Part print with two shaded views. Sizes in mm from the minimum x, y, z corner. A direction names the side the tool comes from. Round coordinates to 2 decimals unless told otherwise and drop trailing zeros. Order: outer loops, then holes, each group sorted by start corner. A loop starts at its lowest first (then second) coordinate and runs counter-clockwise, first axis right, second up. Notation, with made-up numbers: M -40,73 L -9,73 A15 ccw -9,91 Z; hole C -2.5,2 d8. An arc over 180 degrees is marked long. Answer as a JSON object with one key per item and string values.
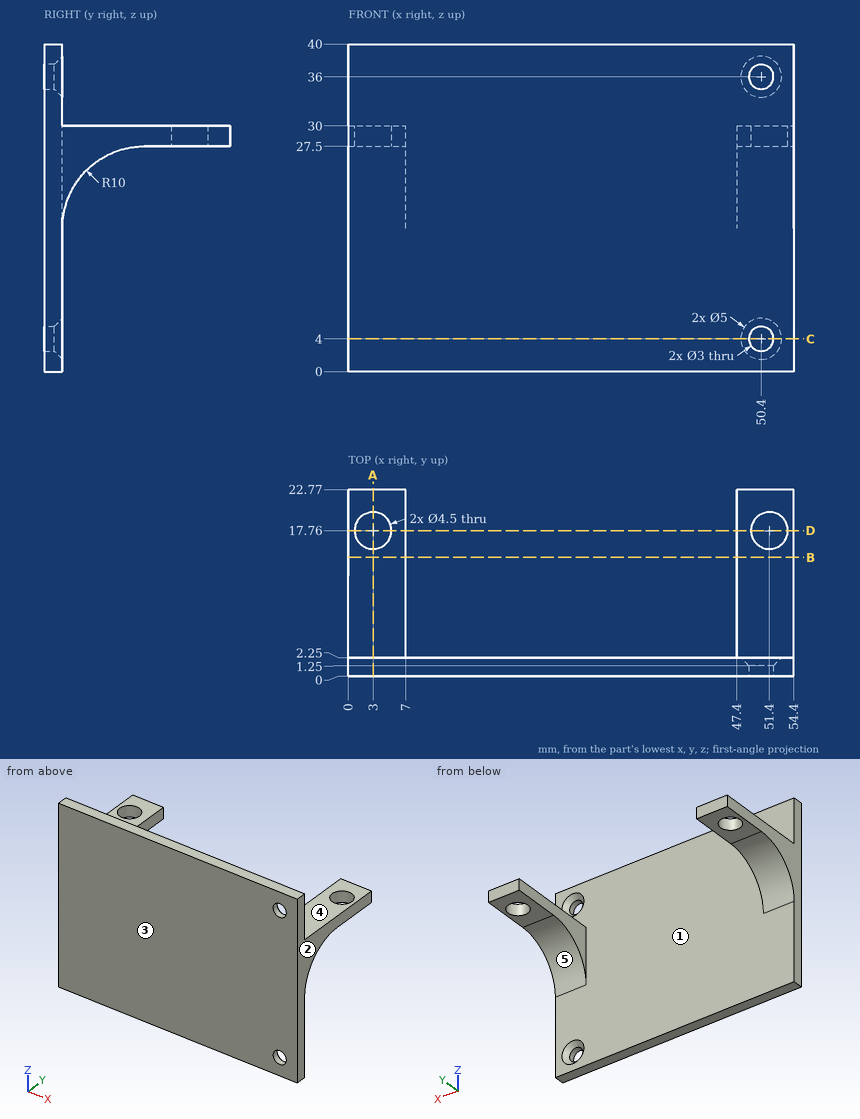
Item 1: 3-axis set-ups, long thin cutter, end or side, ignore diameter. For the marked faces 4 and 5: which of +Z, -Z, +X, -X, +Y, -Y reach the whole face in a straight line?
Worked answers:
{"face 4": "+Z, +X, -X, +Y", "face 5": "-Z, +X, -X, +Y"}
Item 2: Saw through at D-D on y = 17.76. List the corners of the cut face in (x, z), and give its area (3 significant figures).
Worked answers:
{"outline": "M 0,27.5 L 0.75,27.5 L 0.75,30 L 0,30 Z; M 5.25,27.5 L 7,27.5 L 7,30 L 5.25,30 Z; M 47.4,27.5 L 49.15,27.5 L 49.15,30 L 47.4,30 Z; M 53.65,27.5 L 54.4,27.5 L 54.4,30 L 53.65,30 Z", "area": "12.5 mm2"}
Item 3: Saw through at B-B on y = 14.5. List the corners of the cut face in (x, z).
Worked answers:
{"outline": "M 0,27.5 L 7,27.5 L 7,30 L 0,30 Z; M 47.4,27.5 L 54.4,27.5 L 54.4,30 L 47.4,30 Z"}
Item 4: Saw through at C-C on z = 4. List the corners of the cut face in (x, y).
Worked answers:
{"outline": "M 0,0 L 48.9,0 L 48.9,1.25 L 47.9,2.25 L 0,2.25 Z; M 51.9,0 L 54.4,0 L 54.4,2.25 L 52.9,2.25 L 51.9,1.25 Z"}
Item 5: Two-plate mould, pull along X, no slides. Class the marked faces 1, 2 and 3: released by +X, released by -X, zero draft, split by the parting line, or undercut.
Worked answers:
{"face 1": "undercut", "face 2": "released by +X", "face 3": "zero draft"}
Item 6: Drop flat-ended pins along their axis: pin 1 Ø10 at (y, z) = (11.5, 21.5) entering from -X; pin 2 Ø12 at (x, z) = (32.5, 13) entering from +Y; pin 3 Ø7.5 at (x, y) = (3, 14) entering from +Z; pin 4 Ø7.5 at (x, y) = (2, 19) entering from -Z. Give the stop position or say it passes through.
Worked answers:
{"pin 1": "passes through", "pin 2": "stops at y = 2.25", "pin 3": "stops at z = 30", "pin 4": "stops at z = 27.5"}
Item 7: Saw through at A-A on x = 3. List the corners of the cut face in (y, z), and give its area (3 significant figures).
Worked answers:
{"outline": "M 0,0 L 2.25,0 L 2.25,17.5 A10 cw 12.25,27.5 L 15.51,27.5 L 15.51,30 L 2.25,30 L 2.25,40 L 0,40 Z; M 20.01,27.5 L 22.77,27.5 L 22.77,30 L 20.01,30 Z", "area": "152 mm2"}
Item 8: Wall check: line 1 along Y through (x, z) = (3, 28.4); line 2 along X through (y, z) = (1, 4); line 3 along Y through (x, z) = (12.5, 4). Give the ranges that are in metal, low to high. Write a range as [from, to].
Worked answers:
{"line 1": "y = [0, 15.51], [20.01, 22.77]", "line 2": "x = [0, 48.9], [51.9, 54.4]", "line 3": "y = [0, 2.25]"}
